```python
from build123d import *

# Parameters (mm, degrees)
SKETCH_W     = 62
SKETCH_H     = 62
PAD_DEPTH    = 15
FILLET_R     = 7.5
CHAMFER_SIZE = 1
PAD001_DEPTH = 19
FILLET001_R  = 1
SKETCH002_R  = 2
PAD002_DEPTH = 4
SKETCH003_R  = 1.7
PAD003_DEPTH = 6.5
SKETCH004_R  = 2
PAD004_DEPTH = 8
FILLET002_R  = 1.2
FILLET003_R  = 1.2
FILLET004_R  = 1
SKETCH005_R  = 2
PAD005_DEPTH = 15


with BuildPart() as part:
    # Sketch → Pad (new body, symmetric)
    with BuildSketch(Plane.XY):
        Rectangle(SKETCH_W, SKETCH_H)
    extrude(amount=PAD_DEPTH, both=True)

    # Fillet
    fillet_edges = [part.edges().sort_by_distance(p)[0] for p in [
        (31, -31, 0),
        (-31, -31, 0),
        (31, 31, 0),
        (-31, 31, 0),
    ]]
    fillet(fillet_edges, radius=FILLET_R)

    # Chamfer
    chamfer_edges = [part.edges().sort_by_distance(p)[0] for p in [
        (0, 31, 15),
        (-28.803301, 28.803301, 15),
        (-31, 0, 15),
        (31, 0, 15),
        (28.803301, 28.803301, 15),
        (-28.803301, -28.803301, 15),
        (0, -31, 15),
        (28.803301, -28.803301, 15),
        (28.803301, -28.803301, -15),
        (0, -31, -15),
        (-28.803301, -28.803301, -15),
        (-31, 0, -15),
        (31, 0, -15),
        (28.803301, 28.803301, -15),
        (0, 31, -15),
        (-28.803301, 28.803301, -15),
    ]]
    chamfer(chamfer_edges, length=CHAMFER_SIZE)

    # Sketch001 (on Face13 of Chamfer) → Pad001 (join)
    with BuildSketch(Plane.YZ.offset(31)):
        Polygon((6, 11), (6, -11), (12.5, -17), (19, -11), (19, 11), (12.5, 17), align=None)
    extrude(amount=PAD001_DEPTH)

    # Fillet001
    fillet001_edges = [part.edges().sort_by_distance(p)[0] for p in [
        (40.5, 19, 11),
        (40.5, 6, 11),
        (40.5, 12.5, 17),
        (40.5, 6, -11),
        (40.5, 12.5, -17),
        (40.5, 19, -11),
    ]]
    fillet(fillet001_edges, radius=FILLET001_R)

    # Sketch002 (on Face12 of Fillet001) → Pad002 (join)
    with BuildSketch(Plane.YZ.offset(50)):
        with Locations((12.5, 9.5)):
            Circle(SKETCH002_R)
        with Locations((12.5, -9.5)):
            Circle(SKETCH002_R)
    extrude(amount=PAD002_DEPTH)

    # Sketch003 (on Face43 of Pad002) → Pad003 (join)
    with BuildSketch(Plane.YZ.offset(54)):
        with Locations((12.5, 9.5)):
            Circle(SKETCH003_R)
        with Locations((12.5, -9.5)):
            Circle(SKETCH003_R)
    extrude(amount=PAD003_DEPTH)

    # Sketch004 (on Face50 of Pad003) → Pad004 (join)
    with BuildSketch(Plane.YZ.offset(60.5)):
        with Locations((12.5, 9.5)):
            Circle(SKETCH004_R)
        with Locations((12.5, -9.5)):
            Circle(SKETCH004_R)
    extrude(amount=PAD004_DEPTH)

    # Fillet002
    fillet002_edges = [part.edges().sort_by_distance(p)[0] for p in [
        (68.5, 10.5, 9.5),
    ]]
    fillet(fillet002_edges, radius=FILLET002_R)

    # Fillet003
    fillet003_edges = [part.edges().sort_by_distance(p)[0] for p in [
        (68.5, 10.5, -9.5),
    ]]
    fillet(fillet003_edges, radius=FILLET003_R)

    # Cone → Cone (revolve)
    with BuildSketch(Plane(origin=(-31, 0, 0), x_dir=(0, -1, 0), z_dir=(0, 0, -1))):
        Polygon((0, 0), (4, 0), (3, 15), (0, 15), align=None)
    revolve(axis=Axis((-31, 0, 0), (-1, 0, 0)))

    # Fillet004
    fillet004_edges = [part.edges().sort_by_distance(p)[0] for p in [
        (-46, 3, 0),
    ]]
    fillet(fillet004_edges, radius=FILLET004_R)

    # Sketch005 (on Face4 of Fillet004) → Pad005 (join)
    with BuildSketch(Plane(origin=(-46, 0, 0), x_dir=(0, -1, 0), z_dir=(-1, 0, 0))):
        Circle(SKETCH005_R)
    extrude(amount=PAD005_DEPTH)


solid = part.part
```
CAD build for the part. Positions are in the model's coordinates, mm. A direction names the side the tool comes from. Round coordinates to 2 decimals unless told otherwise and drop trailing zeros. Order: outer loops, then holes, each group sorted by start corner. A loop starts at its lowest first (then second) coordinate and runs counter-clockwise, first axis right, second up.
Q1. Slice it at B-B (x = -1.5). Write the cut outline in (y, z).
Q2. Wall check: L1, parallel to X at y = 8, z = 7; L2, parallel to Z at x = 1, y = -0.5; L3, parallel to X at y = 8, z = -14. Give the ranges that are in metal, low to high.
Q3. Two-plate mould, pull along X, no slides. Class faces 1 (the conical face through (28.271, -28.167, 14.826)), 2 (the flat face through (31, 12, 15)), 3 (the flat face through (40, 6, 0)), 4 (the conical face through (-38.13, -3.36, 1.06)): pulls with the +X half, pulls with the -X half, needs draft (parallel to the pull), parting line crosses it, or undercut.
Q4. Which spindle directions (+Z, -Z, +X, -X, +Y, -Y) get a long thin tool onto all of the face, cutting with end or side? Do faces 5 (the flat face through (40.37, 9.11, 13.87)), 6 (the flat face through (40.367, 9.033, -13.8)), 7 (the cylindrical face through (51.972, 11.026, -8.148)), 8 (the cylindrical face through (-53, 0, -2)), 9 (the flat face through (40.367, 15.967, 13.8)). Say none if no direction does.
Q5. Drop flat-ended pins along their axis: pin 1 (15 mm diameter, centred on x = 39, z = 3.5, fed in from +Y); pin 2 (5 mm diameter, centred on y = 17.5, z = -6, fed in from +X); pin 3 (4.5 mm diameter, centred on y = 13, z = 9.5, fed in from -X). Give the stop position or say it passes through.
Q6. Slice it at A-A (y = 0). Write the cut outline in (x, z), and give its area (3 significant figures).
Q7. Slice it at C-C (z = 0). Write the cut outline in (x, y).
Results below:
1. outline: (-31, -14) - (-30, -15) - (30, -15) - (31, -14) - (31, 14) - (30, 15) - (-30, 15) - (-31, 14) - close
2. L1: x = -31 to 50
2. L2: z = -15 to 15
2. L3: x = -31 to 31
3. face 1: pulls with the +X half
3. face 2: undercut
3. face 3: needs draft
3. face 4: pulls with the -X half
4. face 5: +Z, +X, -Y
4. face 6: -Z, +X, -Y
4. face 7: +X
4. face 8: -X
4. face 9: +Z, +X, +Y
5. pin 1: stops at y = 19
5. pin 2: stops at x = 50
5. pin 3: stops at x = -31
6. outline: (-61, -2) - (-46, -2) - (-46, -2.06) arc R1 ccw to (-45.07, -3.06) - (-31, -4) - (-31, -14) - (-30, -15) - (30, -15) - (31, -14) - (31, 14) - (30, 15) - (-30, 15) - (-31, 14) - (-31, 4) - (-45.07, 3.06) arc R1 ccw to (-46, 2.06) - (-46, 2) - (-61, 2) - close
6. area: 2,020 mm2
7. outline: (-61, -2) - (-46, -2) - (-46, -2.06) arc R1 ccw to (-45.07, -3.06) - (-31, -4) - (-31, -23.5) arc R7.5 ccw to (-23.5, -31) - (23.5, -31) arc R7.5 ccw to (31, -23.5) - (31, 6) - (50, 6) - (50, 19) - (31, 19) - (31, 23.5) arc R7.5 ccw to (23.5, 31) - (-23.5, 31) arc R7.5 ccw to (-31, 23.5) - (-31, 4) - (-45.07, 3.06) arc R1 ccw to (-46, 2.06) - (-46, 2) - (-61, 2) - close
